Could you check a few things on this model? Use its own coordinates, in mm. Round coordinates to 2 decimals unless told otherwise and drop trailing zeros. Loops run counter-clockwise (first coordinate to the right, second up) from the corner with the lowest first, then second, coordinate; pieces in that order, holes last. Notation, with made-up numbers: (32.5, -4) -> (53.5, -4) arc R14 cw to (53.5, 23) -> close; hole circle Ø2 at (0.25, -31.5). An arc over 180 degrees is marked (long way). Put each result on its own line as item: value. Start each with the question number.
1. Imagine slicing it at A-A, the plane y = -6. Please give me the cut outline in (x, z), and give its area (3 significant figures).
2. Imagine slicing it at C-C, the plane z = -22.5. Please give me the cut outline in (x, y).
3. Imagine slicing it at D-D, the plane z = 24.5. Count the separate pieces of the cut face and the enclosed holes in it, and give its area (3 significant figures).
4. Imagine slicing it at B-B, the plane z = 0. Please give me the cut outline in (x, y).
5. If we mould it in two halves opening along X, with no side actions, what happens to faces 1 (the flat face through (0, -6, -35)), 2 (the cylindrical face through (17.269, -6.077, -27.745)), 3 (the flat face through (-35, -6, 0))? For each: pulls with the +X half, pulls with the -X half, needs draft (parallel to the pull), parting line crosses it, or undercut.
6. I need wall thicknesses on line 1 (X direction, y = -5.5, z = -22.5); line 2 (X direction, y = -4.75, z = 22.5); line 3 (Z direction, x = 0, y = -9). Which ranges of each line are inside material? Lowest first, please. Write a range as [from, to].
Autodesk Inventor part; units mm, degrees
ref_plane "YZ Plane" through (0, 0, 0) normal (1, 0, 0) x (0, 1, 0)
ref_plane "XZ Plane" through (0, 0, 0) normal (0, 1, 0) x (-1, 0, 0)
ref_plane "XY Plane" through (0, 0, 0) normal (0, 0, 1) x (1, 0, 0)
sketch "Sketch1" plane through (0, 0, 0) normal (0, 1, 0) x (-1, 0, 0)
  line L0 (-35, 35) -> (35, 35)
  line L1 (35, 35) -> (35, -35)
  line L2 (35, -35) -> (-35, -35)
  line L3 (-35, -35) -> (-35, 35)
  line L4 (-35, 35) -> (35, -35) construction
  line L5 (35, 35) -> (-35, -35) construction
  line L6 (-22.5, 22.5) -> (22.5, 22.5) construction
  line L7 (22.5, 22.5) -> (22.5, -22.5) construction
  line L8 (22.5, -22.5) -> (-22.5, -22.5) construction
  line L9 (-22.5, -22.5) -> (-22.5, 22.5) construction
  line L10 (-22.5, 22.5) -> (22.5, -22.5) construction
  line L11 (22.5, 22.5) -> (-22.5, -22.5) construction
  line L12 (-17.5, 22.5) -> (17.5, 22.5) construction
  line L13 (17.5, 22.5) -> (17.5, -22.5) construction
  line L14 (17.5, -22.5) -> (-17.5, -22.5) construction
  line L15 (-17.5, -22.5) -> (-17.5, 22.5) construction
  line L16 (-17.5, 22.5) -> (17.5, -22.5) construction
  line L17 (17.5, 22.5) -> (-17.5, -22.5) construction
  circle A0 centre (0, 0) radius 7
  dimension "d0" = 70
  dimension "d1" = 45
  dimension "d2" = 35
  dimension "d3" = 14
  dimension "d16" = 70
  dimension "d17" = 45
extrude "Extrusion1" add sketch "Sketch1" against normal blind 12
hole "Hole1" at (-17.5, 0, -22.5) at (17.5, 0, -22.5) at (-22.5, 0, 22.5) at (22.5, 0, 22.5) direction (0, -1, 0) diameter 10.5 end through all
chamfer "Chamfer1" distance 0.5 angle 45 10 edges at (17.5, 0, -27.75) (-17.5, 0, -27.75) (22.5, 0, 17.25) (-22.5, 0, 17.25) (17.5, -12, -27.75) (-17.5, -12, -27.75) (22.5, -12, 17.25) (-22.5, -12, 17.25) (7, 0, 0) (7, -12, 0)
chamfer "Chamfer2" distance 1 angle 45 4 edges at (-35, -6, -35) (35, -6, -35) (35, -6, 35) (-35, -6, 35)
properties part number "AP1-002"
Entries:
1. outline: (-35, -34) -> (-34, -35) -> (34, -35) -> (35, -34) -> (35, 34) -> (34, 35) -> (-34, 35) -> (-35, 34) -> close; hole circle Ø10.5 at (-22.5, 22.5); hole circle Ø10.5 at (-17.5, -22.5); hole circle Ø14 at (0, 0); hole circle Ø10.5 at (17.5, -22.5); hole circle Ø10.5 at (22.5, 22.5)
1. area: 4,400 mm^2
2. outline: (-35, -12) -> (-23.25, -12) -> (-22.75, -11.5) -> (-22.75, -0.5) -> (-23.25, 0) -> (-35, 0) -> close; (-12.25, -11.5) -> (-11.75, -12) -> (11.75, -12) -> (12.25, -11.5) -> (12.25, -0.5) -> (11.75, 0) -> (-11.75, 0) -> (-12.25, -0.5) -> close; (22.75, -11.5) -> (23.25, -12) -> (35, -12) -> (35, 0) -> (23.25, 0) -> (22.75, -0.5) -> close
3. separate pieces: 3
3. enclosed holes: 0
3. area: 606 mm^2
4. outline: (-35, -12) -> (-7.5, -12) -> (-7, -11.5) -> (-7, -0.5) -> (-7.5, 0) -> (-35, 0) -> close; (7, -11.5) -> (7.5, -12) -> (35, -12) -> (35, 0) -> (7.5, 0) -> (7, -0.5) -> close
5. face 1: needs draft
5. face 2: undercut
5. face 3: pulls with the -X half
6. line 1: [-35, -22.75], [-12.25, 12.25], [22.75, 35]
6. line 2: [-35, -27.75], [-17.25, 17.25], [27.75, 35]
6. line 3: [-35, -7], [7, 35]
